Autodesk Fusion 360 part; units mm, degrees
sketch "スケッチ1" plane through (0, 0, 0) normal (0, 0, 1) x (1, 0, 0)
  line L0 (125, -60) -> (-125, -60)
  line L1 (-125, -60) -> (-125, 60)
  line L2 (-125, 60) -> (125, 60)
  line L3 (125, 60) -> (125, -60)
  line L4 (125, -60) -> (-125, 60) construction
  line L5 (-125, -60) -> (125, 60) construction
  dimension "d1" = 250
  dimension "d2" = 120
extrude "押し出し1" add sketch "スケッチ1" along normal blind 120
sketch "スケッチ2" plane through (0, 0, 120) normal (0, 0, 1) x (-1, 0, 0)
  line L0 (-125, -60) -> (125, -60)
  line L1 (125, -60) -> (125, 60)
  line L2 (125, 60) -> (-125, 60)
  line L3 (-125, 60) -> (-125, -60)
  line L4 (-125, 55) -> (125, 55)
  line L5 (125, 55) -> (125, -55)
  line L6 (125, -55) -> (-125, -55)
  line L7 (-125, -55) -> (-125, 55)
  line L8 (-125, 55) -> (125, -55) construction
  line L9 (125, 55) -> (-125, -55) construction
  dimension "d5" = 250
  dimension "d6" = 110
extrude "押し出し2" cut sketch "スケッチ2" against normal blind 115 contours L1 L3 L4 L5 L6 L7
sketch "スケッチ3" plane through (0, 0, 5) normal (0, 0, 1) x (-1, 0, 0)
  line L0 (-125, -55) -> (125, -55)
  line L1 (125, -55) -> (125, 55)
  line L2 (125, 55) -> (-125, 55)
  line L3 (-125, 55) -> (-125, -55)
  line L4 (-125, -55) -> (-120, -55)
  line L5 (-120, -55) -> (-120, 55)
  line L6 (-120, 55) -> (-125, 55)
  line L7 (-125, 55) -> (-125, -55)
extrude "押し出し3" add sketch "スケッチ3" along normal blind 50 contours L0 L2 L3 L4 L5 L6 L7
sketch "スケッチ4" plane through (0, 0, 5) normal (0, 0, 1) x (-1, 0, 0)
  line L0 (-120, 55) -> (-120, -55)
  line L1 (-120, -55) -> (125, -55)
  line L2 (125, -55) -> (125, 55)
  line L3 (125, 55) -> (-120, 55)
  line L4 (120, -55) -> (125, -55)
  line L5 (125, -55) -> (125, 55)
  line L6 (125, 55) -> (120, 55)
  line L7 (120, 55) -> (120, -55)
extrude "押し出し4" add sketch "スケッチ4" along normal blind 30 contours L1 L2 L3 L4 L5 L6 L7
Source: CAD feature listing. Evaluate the final solid. Frame: model axes, mm. A direction names the side the tool comes from. Round coordinates to 2 decimals unless told otherwise and drop trailing zeros. Loops run counter-clockwise (first coordinate to the right, second up) from the corner with the lowest first, then second, coordinate; pieces in that order, holes last.
Q1. Section A-A, the plane z = 20. Return loops of the section in (x, y).
Q2. Section C-C, the plane z = 101. Return loops of the section in (x, y), plus the area to 3 significant figures.
Q3. Access query for faces 4 (the face through (-2, 55, 63)), 5 (the face through (-122, -1, 35)), 6 (the face through (123, -1, 55)), 7 (the face through (-2, 60, 59)). Directions: +Z, -Z, +X, -X, +Y, -Y. A direction counts if a zero-diameter tool reaches every point of the face in a straight line with its end or side. Return the directions, or none.
Q4. Section D-D, the plane x = -81. Return loops of the section in (y, z).
Q5. Ray query, line 1 (Y direction, x = -113, z = 23); line 2 (X direction, y = -22.5, z = 34.5); line 3 (Z direction, x = 40.5, y = 51). Return the intervals inside material, ascending.
Q6. Mould query, pull axis X, two halves, no side actions, for faces 1 (the face through (-120, -1, 20)), 2 (the face through (125, -1, 19)), 3 (the face through (-2, -57, 120)). Classes: pulls with the +X half, pulls with the -X half, needs draft (parallel to the pull), parting line crosses it, or undercut.
Q7. First-contact query: P1, Ø1.5, axis at x = -16, y = 21, coming from the -Z side; P2, Ø1.5, axis at x = -123, y = -7, coming from the +Z side; P3, Ø4, axis at x = 82, y = 27, coming from the +Z side; P4, Ø5.5, axis at x = 123, y = 2, coming from the +Z side. Flat tips, straight axial feed; report the tip coordinate or a pass-through.
Q8. Section B-B, the plane y = 26.5. Return loops of the section in (x, z), plus the area to 3 significant figures.
Solutions:
1. outline: (-125, -60) - (125, -60) - (125, 60) - (-125, 60) - close; hole (-120, -55) - (120, -55) - (120, 55) - (-120, 55) - close
2. outline: (-125, -60) - (125, -60) - (125, -55) - (-125, -55) - close; (-125, 55) - (125, 55) - (125, 60) - (-125, 60) - close
2. area: 2,500 mm2
3. face 4: +Z
3. face 5: +Z, -X
3. face 6: +Z, +X, -X
3. face 7: +Z, -Z, +X, -X, +Y
4. outline: (-60, 0) - (60, 0) - (60, 120) - (55, 120) - (55, 5) - (-55, 5) - (-55, 120) - (-60, 120) - close
5. line 1: y = -60 to -55, 55 to 60
5. line 2: x = -125 to -120, 120 to 125
5. line 3: z = 0 to 5
6. face 1: undercut
6. face 2: pulls with the +X half
6. face 3: needs draft
7. P1: stops at z = 0
7. P2: stops at z = 35
7. P3: stops at z = 5
7. P4: stops at z = 55
8. outline: (-125, 0) - (125, 0) - (125, 55) - (120, 55) - (120, 5) - (-120, 5) - (-120, 35) - (-125, 35) - close
8. area: 1,650 mm2
